from build123d import *

# Parameters (mm, degrees)
CROQUIS1_W              = 68.32
CROQUIS1_H              = 150
CROQUIS1_R              = 1.8
SALIENTE_EXTRUIR1_DEPTH = 2
CROQUIS2_W              = 3
CROQUIS2_H              = 150
SALIENTE_EXTRUIR2_DEPTH = 45
CROQUIS3_W              = 3
CROQUIS3_H              = 150
SALIENTE_EXTRUIR3_DEPTH = 45
CROQUIS4_R              = 6
CROQUIS4_R_2            = 1.9
CORTAR_EXTRUIR1_DEPTH   = 112.810654233
MATRIZC1_COUNT          = 4


with BuildPart() as part:
    # Croquis1 → Saliente-Extruir1 (new body)
    with BuildSketch(Plane(origin=(0, 0, 0), x_dir=(1, 0, 0), z_dir=(0, 1, 0))):
        Rectangle(CROQUIS1_W, CROQUIS1_H)
        with Locations(Location((24.16, 45.2, 0), (0, 0, 270))):
            Circle(CROQUIS1_R, mode=Mode.SUBTRACT)
        with Locations(Location((24.16, 55.2, 0), (0, 0, 270))):
            Circle(CROQUIS1_R, mode=Mode.SUBTRACT)
        with Locations(Location((-24.16, -55.2, 0), (0, 0, 90))):
            Circle(CROQUIS1_R, mode=Mode.SUBTRACT)
        with Locations(Location((24.16, -55.2, 0), (0, 0, 90))):
            Circle(CROQUIS1_R, mode=Mode.SUBTRACT)
        with Locations(Location((-24.16, 45.2, 0), (0, 0, 270))):
            Circle(CROQUIS1_R, mode=Mode.SUBTRACT)
        with Locations(Location((-24.16, 55.2, 0), (0, 0, 270))):
            Circle(CROQUIS1_R, mode=Mode.SUBTRACT)
        with Locations(Location((-24.16, -45.2, 0), (0, 0, 90))):
            Circle(CROQUIS1_R, mode=Mode.SUBTRACT)
        with Locations(Location((24.16, -45.2, 0), (0, 0, 90))):
            Circle(CROQUIS1_R, mode=Mode.SUBTRACT)
    extrude(amount=SALIENTE_EXTRUIR1_DEPTH)

    # Croquis2 → Saliente-Extruir2 (add)
    with BuildSketch(Plane(origin=(0, 2, 0), x_dir=(1, 0, 0), z_dir=(0, 1, 0))):
        with Locations((-32.66, 0)):
            Rectangle(CROQUIS2_W, CROQUIS2_H)
    extrude(amount=SALIENTE_EXTRUIR2_DEPTH)

    # Croquis3 → Saliente-Extruir3 (add)
    with BuildSketch(Plane(origin=(0, 2, 0), x_dir=(1, 0, 0), z_dir=(0, 1, 0))):
        with Locations((32.66, 0)):
            Rectangle(CROQUIS3_W, CROQUIS3_H)
    extrude(amount=SALIENTE_EXTRUIR3_DEPTH)

    # Croquis4 → Cortar-Extruir1 (cut, through all)
    with BuildSketch(Plane.ZY.offset(34.16)):
        with Locations((0, 23.5)):
            Circle(CROQUIS4_R)
        with Locations((7.071067812, 30.571067812)):
            Circle(CROQUIS4_R_2)
    cortar_extruir1 = extrude(amount=-CORTAR_EXTRUIR1_DEPTH, mode=Mode.SUBTRACT)

    # MatrizC1: Cortar-Extruir1 ×4 about axis
    matrizc1_axis = Axis((0, 23.5, 0), (1, 0, 0))
    for i in range(1, MATRIZC1_COUNT):
        add(cortar_extruir1.rotate(matrizc1_axis, i * 360 / MATRIZC1_COUNT), mode=Mode.SUBTRACT)


solid = part.part
The model under review builds one solid part; all positions refer to its coordinate system, in mm. A direction names the side the tool comes from. Round coordinates to 2 decimals unless told otherwise and drop trailing zeros. Loops run counter-clockwise (first coordinate to the right, second up) from the corner with the lowest first, then second, coordinate; pieces in that order, holes last. Notation, with made-up numbers: M -5,35 L 44,35 A10 cw 44,39 Z; hole C 15.25,43 d8. An arc over 180 degrees is marked long. Answer as CSV lines item,"result".
1. To check wall thickness, follow L1, parallel to X at y = 0.8, z = -55.2; L2, parallel to X at y = 1, z = -55; L3, parallel to X at y = 30, z = 27. State the ranges of each line that lie inside material, in increasing order. Write a range as [from, to].
Outcome:
L1,"x = [-34.16, -25.96], [-22.36, 22.36], [25.96, 34.16]"
L2,"x = [-34.16, -25.95], [-22.37, 22.37], [25.95, 34.16]"
L3,"x = [-34.16, -31.16], [31.16, 34.16]"
2. We need section D-D (z = 22.5). Give the boundary of the cut face in (x, y).
Outcome:
outline,"M -34.16,0 L 34.16,0 L 34.16,47 L 31.16,47 L 31.16,2 L -31.16,2 L -31.16,47 L -34.16,47 Z"
3. Insertion check: pin 1 Ø2.5 at (y, z) = (30.57, 7.07) entering from +X (1 decimal); pin 2 Ø18.5 at (x, z) = (-7, -18.5) entering from +Y. Each pin has a flat end and moves straight along its axis. Give the tip position at first contact, or say it passes through.
Outcome:
pin 1,"passes through"
pin 2,"stops at y = 2"
4. We need section B-B (x = -24.16). Give the boundary of the cut face in (y, z), plus the area to 3 significant figures.
Outcome:
outline,"M 0,-75 L 2,-75 L 2,-57 L 0,-57 Z; M 0,-53.4 L 2,-53.4 L 2,-47 L 0,-47 Z; M 0,-43.4 L 2,-43.4 L 2,43.4 L 0,43.4 Z; M 0,47 L 2,47 L 2,53.4 L 0,53.4 Z; M 0,57 L 2,57 L 2,75 L 0,75 Z"
area,"271 mm2"
5. We need section A-A (z = 45.2). Give the boundary of the cut face in (x, y).
Outcome:
outline,"M -34.16,0 L -25.96,0 L -25.96,2 L -31.16,2 L -31.16,47 L -34.16,47 Z; M -22.36,0 L 22.36,0 L 22.36,2 L -22.36,2 Z; M 25.96,0 L 34.16,0 L 34.16,47 L 31.16,47 L 31.16,2 L 25.96,2 Z"
6. We need section C-C (y = 27). Give the boundary of the cut face in (x, z).
Outcome:
outline,"M -34.16,-75 L -31.16,-75 L -31.16,-4.87 L -34.16,-4.87 Z; M -34.16,4.87 L -31.16,4.87 L -31.16,75 L -34.16,75 Z; M 31.16,-75 L 34.16,-75 L 34.16,-4.87 L 31.16,-4.87 Z; M 31.16,4.87 L 34.16,4.87 L 34.16,75 L 31.16,75 Z"
7. For faces 4 (the face through (0, 2, -1)), 5 (the face through (32.639, 14.617, 7.642)), list the 3-axis set-ups (+Z, -Z, +X, -X, +Y, -Y) from which the entire face can be reached by the end or side of a thin tool; tool diameter is ignored.
Outcome:
face 4,"+Z, -Z, +Y"
face 5,"+X, -X"
8. Draft analysis for pull direction Z (two halves, no side actions). For faces 1 (the face through (31.16, 14, 1)), 2 (the face through (-32.681, 18.115, -7.948)), 3 (the face through (0, 1, -75)), state which applies: pulls with the +Z half, pulls with the -Z half, needs draft (parallel to the pull), parting line crosses it, or undercut.
Outcome:
face 1,"needs draft"
face 2,"undercut"
face 3,"pulls with the -Z half"
